Geometry check sheet. Reference: the model listing, model coordinates, mm. A direction names the side the tool comes from. Coordinates: 2 decimals unless noted, no trailing zeros. Loops run counter-clockwise (first coordinate to the right, second up) from the corner with the lowest first, then second, coordinate; pieces in that order, holes last.
Autodesk Inventor part; units mm, degrees
ref_plane "C_XY" through (3, 0, 0) normal (1, 0, 0) x (0, 0, -1)
ref_plane "C_YZ" through (3, 0, 0) normal (0, 0, -1) x (0, 1, 0)
ref_plane "C_ZX" through (3, 0, 0) normal (0, 1, 0) x (1, 0, 0)
sketch "Sketch_1" plane through (0, 0, 0) normal (0, 0, 1) x (1, 0, 0)
  line L0 (6, 0) -> (0, 0)
  line L1 (0, 8.75) -> (0, 3.6)
  line L2 (0, 3.6) -> (6, 3.6)
  line L3 (6, 3.6) -> (6, 8.75)
  line L4 (6, 8.75) -> (0, 8.75)
revolve "Revolution1" add sketch "Sketch_1" angle 360 about axis through (6, 0, 0) along (1, 0, 0)
sketch "Sketch_2" plane through (0, 0, 0) normal (0, 0, 1) x (1, 0, 0)
  line L0 (0, -2.3) -> (2.9, -2.3)
  line L1 (2.9, -2.3) -> (2.9, 2.3)
  line L2 (2.9, 2.3) -> (0, 2.3)
  line L3 (0, 2.3) -> (0, -2.3)
extrude "Extrusion1" cut sketch "Sketch_2" along normal mid plane 17.5
sketch "Sketch_3" plane through (0, 0, 0) normal (0, 1, 0) x (-1, 0, 0)
  line L0 (-3.1, -2.3) -> (-3.1, 2.3)
  line L1 (-3.1, 2.3) -> (-6, 2.3)
  line L2 (-6, 2.3) -> (-6, -2.3)
  line L3 (-6, -2.3) -> (-3.1, -2.3)
extrude "Extrusion2" cut sketch "Sketch_3" along normal mid plane 17.5
ref_plane "C_XY" through (3, 0, 0) normal (1, 0, 0) x (0, 0, -1)
ref_plane "C_YZ" through (3, 0, 0) normal (0, 0, -1) x (0, 1, 0)
ref_plane "C_ZX" through (3, 0, 0) normal (0, 1, 0) x (1, 0, 0)
properties part number "MCOC_spacer17"
1) Section check D-D on y = -6.5. Record the cut outline in (x, z), and give its area (3 significant figures).
Data:
outline: (0, -5.86) - (6, -5.86) - (6, -2.3) - (3.1, -2.3) - (3.1, 2.3) - (6, 2.3) - (6, 5.86) - (0, 5.86) - close
area: 57.0 mm2
2) Mould release check, pull along Y, two halves, no side actions. Record for faces 1 (the cylindrical face through (2.958, 8.083, 3.351)), 2 (the cylindrical face through (3.042, -2.653, 2.433)), 3 (the flat face through (0, 5, 0)): +Y half, -Y half, draft (parallel to the pull), parting line (faces both ways), or undercut.
Data:
face 1: parting line
face 2: undercut
face 3: draft
3) Section check C-C on z = 5.75. Record the cut outline in (x, y).
Data:
outline: (0, -6.6) - (6, -6.6) - (6, 6.6) - (0, 6.6) - (0, 2.3) - (2.9, 2.3) - (2.9, -2.3) - (0, -2.3) - close
4) Access from +Z, -Z, +X, -X, +Y, -Y to the whole of each face (thin tool, end or side, straight path). Record for faces 4 (the flat face through (1, 2.3, -6)), 5 (the flat face through (6, 0, 5)), 6 (the flat face through (5, 6, -2.3)).
Data:
face 4: +Z, -Z, -X
face 5: +Z, -Z, +X, +Y, -Y
face 6: +X, +Y, -Y
5) Material ranges on probe 1 along Z at (x, y) = (4.8, 0); probe 2 along X at (y, z) = (6.5, 0.25); probe 3 along Y at (x, z) = (2, -2.5), recorded low to high.
Data:
probe 1: z = -8.75 to -3.6, 3.6 to 8.75
probe 2: x = 0 to 3.1
probe 3: y = -8.39 to -2.59, 2.59 to 8.39
6) Section check B-B on z = 0. Record the cut outline in (x, y), and give its area (3 significant figures).
Data:
outline: (0, -8.75) - (3.1, -8.75) - (3.1, -3.6) - (0, -3.6) - close; (0, 3.6) - (3.1, 3.6) - (3.1, 8.75) - (0, 8.75) - close
area: 31.9 mm2
7) Depth check by flat-ended pin: pin 1 (3 mm diameter, centred on x = 1, z = 6.5, fed in from +Y); pin 2 (2.5 mm diameter, centred on y = 6.5, z = -0.5, fed in from +X); pin 3 (3.5 mm diameter, centred on y = -6.5, z = 1, fed in from +X); pin 4 (6 mm diameter, centred on y = 0, z = 0, fed in from -X). Enter the tip coordinate at first touch or a pass-through.
Data:
pin 1: stops at y = 7.18
pin 2: stops at x = 3.1
pin 3: stops at x = 6
pin 4: passes through
8) Section check A-A on y = 0. Record the cut outline in (x, z).
Data:
outline: (2.9, -8.75) - (6, -8.75) - (6, -3.6) - (2.9, -3.6) - close; (2.9, 3.6) - (6, 3.6) - (6, 8.75) - (2.9, 8.75) - close
